Input: part model. Units: mm. Frame: model coordinates. Face numbers are marked on the shaded views. A direction names the side the tool comes from. Give positions to 0.01 mm unless a question says otherwise; leave off trailing zeros. Order: outer loops, then holes, each group sorted by start corner. A loop starts at its lowest first (then second) coordinate and runs counter-clockwise, first axis right, second up.
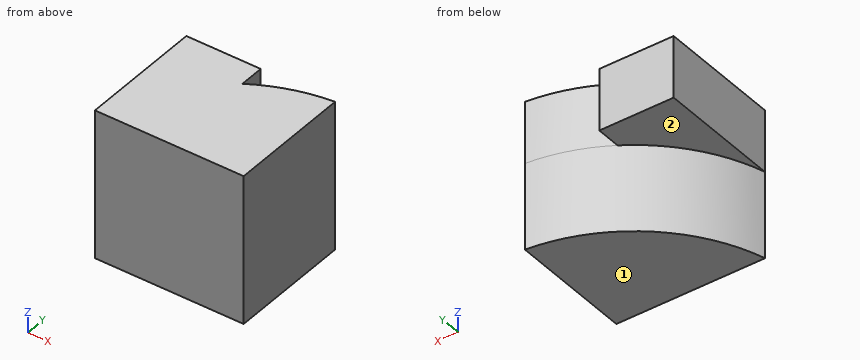
```python
from build123d import *

# Parameters (mm, degrees)
SKETCH1_W           = 6
SKETCH1_H           = 6
BOSS_EXTRUDE1_DEPTH = 5
CUT_EXTRUDE12_DEPTH = 3.5
CUT_EXTRUDE13_DEPTH = 3.5


with BuildPart() as part:
    # Sketch1 → Boss-Extrude1 (new body)
    with BuildSketch(Plane(origin=(0, 0, 0), x_dir=(1, 0, 0), z_dir=(0, 1, 0))):
        Rectangle(SKETCH1_W, SKETCH1_H)
    extrude(amount=BOSS_EXTRUDE1_DEPTH)

    # Sketch13 → Cut-Extrude12 (cut)
    with BuildSketch(Plane(origin=(0, 0, -3), x_dir=(-1, 0, 0), z_dir=(0, 0, -1))):
        with BuildLine():
            ThreePointArc((-3, 5), (0.780941195, 3.437129434), (3, 0))
            Line((3, 0), (3, 5))
            Line((3, 5), (-3, 5))
        make_face()
    extrude(amount=-CUT_EXTRUDE12_DEPTH, mode=Mode.SUBTRACT)

    # Sketch14 → Cut-Extrude13 (cut)
    with BuildSketch(Plane(origin=(0, 0, 0.5), x_dir=(-1, 0, 0), z_dir=(0, 0, -1))):
        with BuildLine():
            ThreePointArc((-3, 5), (-1.441597312, 4.675208063), (0, 4))
            Line((0, 4), (0, 5))
            Line((0, 5), (-3, 5))
        make_face()
    extrude(amount=-CUT_EXTRUDE13_DEPTH, mode=Mode.SUBTRACT)


solid = part.part
```
1) Cut plane B-B (z = 2.1). Return the cut outline in (x, y).
2) Line query: probe 1 along X at (y, z) = (4, -0.6); probe 2 along X at (y, z) = (4.3, 0.55); probe 3 along X at (y, z) = (4.45, 2.1). Output: solid intervals per line, ascending.
3) Reachability of the marked faces 1 and 2 from +Z, -Z, +X, -X, +Y, -Y: full face, straight path, thin tool, end or side. Return the list, or none.
4) Cut plane C-C (x = 1.5). Return the cut outline in (y, z).
5) Cut plane D-D (y = 3.9). Return the cut outline in (x, z), then the cut area to 3 significant figures.
6) Cut plane A-A (y = 4.5). Return the cut outline in (x, z), then the cut area to 3 significant figures.
7) First-contact query: P1, Ø2, axis at x = 0.5, z = 2, coming from the +Y side. Flat tip, straight axial feed; report the tip coordinate or a pass-through.
Geometry says:
1. outline: (-3, 0) - (3, 0) - (3, 5) arc R6.86 ccw to (0, 4) - (0, 5) - (-3, 5) - close
2. probe 1: x = 0 to 3
2. probe 2: x = -3 to 0, 0.54 to 3
2. probe 3: x = -3 to 0, 0.86 to 3
3. face 1: -Z, +X, -X, +Y, -Y
3. face 2: -Z, -X, +Y
4. outline: (0, -3) - (4.69, -3) - (4.69, 3) - (0, 3) - close
5. outline: (-3, 0.5) - (-0.16, 0.5) - (-0.16, -3) - (3, -3) - (3, 3) - (-3, 3) - close
5. area: 26.0 mm2
6. outline: (-3, 0.5) - (0, 0.5) - (0, 3) - (-3, 3) - close; (0.97, -3) - (3, -3) - (3, 3) - (0.97, 3) - close
6. area: 19.7 mm2
7. P1: stops at y = 5
